from build123d import *

# Parameters (mm, degrees)
BOSS_EXTRUDE1_DEPTH = 17
M8_TAPPED_HOLE1_D   = 6.8


with BuildPart() as part:
    # Sketch1 → Boss-Extrude1 (new body)
    with BuildSketch(Plane(origin=(0, 0, 0), x_dir=(1, 0, 0), z_dir=(0, 1, 0))):
        with BuildLine():
            Line((10.214282758, -18.266545266), (13.128495977, -15.352332485))
            ThreePointArc((13.128495977, -15.352332485), (13.345268844, -15.027908548), (13.421388977, -14.645224485))
            Line((13.421388977, -14.645224485), (13.421388977, -5.451641485))
            ThreePointArc((13.421388977, -5.451641485), (13.345268461, -5.068958498), (13.128495977, -4.744535485))
            Line((13.128495977, -4.744535485), (10.214282758, -1.830320704))
            ThreePointArc((10.214282758, -1.830320704), (9.889859409, -1.613547953), (9.507175977, -1.537427485))
            Line((9.507175977, -1.537427485), (8.421388977, -1.537427485))
            ThreePointArc((8.421388977, -1.537427485), (7.714282177, -1.830320722), (7.421388977, -2.537427537))
            Line((7.421388977, -2.537427537), (7.421388977, -5.159438485))
            Line((7.421388977, -5.159438485), (4.421388977, -5.159438485))
            Line((4.421388977, -5.159438485), (4.421388977, -14.959438485))
            Line((4.421388977, -14.959438485), (7.421388977, -14.959438485))
            Line((7.421388977, -14.959438485), (7.421388977, -17.559438537))
            ThreePointArc((7.421388977, -17.559438537), (7.714282276, -18.266545347), (8.421389151, -18.559438485))
            Line((8.421389151, -18.559438485), (9.507176151, -18.559438485))
            ThreePointArc((9.507176151, -18.559438485), (9.88985949, -18.483317984), (10.214282758, -18.266545266))
        make_face()
    extrude(amount=BOSS_EXTRUDE1_DEPTH)

    # M8 Tapped Hole1 (through all)
    with Locations(Plane(origin=(4.421388977, 8.5, 10.059438485), x_dir=(0, 0, -1), z_dir=(-1, 0, 0))):
        with Locations((0, 0)):
            Hole(M8_TAPPED_HOLE1_D / 2)


solid = part.part
Design review of the part built by this model. Coordinates are the model's own, in mm. A direction names the side the tool comes from. Round coordinates to 2 decimals unless told otherwise and drop trailing zeros. Write each loop counter-clockwise with the first axis right and the second up, starting at its lowest first coordinate (ties: lowest second). Pieces come first, ordered by that corner, then holes. Notation, with made-up numbers: (10, -2.5) - (28, -2.5) arc R6 ccw to (28, 6.5) - close; hole circle Ø8 at (59.5, 31). An arc over 180 degrees is marked (long way). Use a Markdown table: item, result. Add a question column.
1. Clearance check with flat-ended pins moving along their axes: pin 1 (2 mm diameter, centred on y = 7, z = 4.5, fed in from -X); pin 2 (0.8 mm diameter, centred on y = 5, z = 16, fed in from -X); pin 3 (1.5 mm diameter, centred on x = 12.5, y = 8, fed in from -Z); pin 4 (1.5 mm diameter, centred on x = 6, y = 12, fed in from -Z). State where each tip first meets the part, or that it passes through.
2. We need section A-A (y = 8.5). State the section outline as (x, z) points, then the cut area to 3 significant figures.
3. We need section D-D (y = 12.75). State the section outline as (x, z) points.
4. For faces 1 (the face through (7.421, 8, 16)), 2 (the face through (7.421, 8, 4)), 3 (the face through (9, 8, 1.537)), list the 3-axis set-ups (+Z, -Z, +X, -X, +Y, -Y) from which the entire face can be reached by the end or side of a thin tool; tool diameter is ignored.
5. We need section B-B (x = 5.5). State the section outline as (y, z) points.
6. Wall thickness on probe 1 along Z at (x, y) = (6.75, 8.5); probe 2 along Z at (x, y) = (9.25, 8.5); probe 3 along Y at (x, z) = (11, 12.75): over which ranges is each line inside the solid? List them lowest first.
7. Mouldability with a two-part tool opening along Y and no side actions: class faces 4 (the face through (9, 9.8, 13.2)), 5 (the face through (9, 17, 10)), 6 (the face through (9, 0, 10)), 7 (the face through (11.65, 8.38, 16.83)) as +Y half, -Y half, draft (parallel to the pull), parting line (faces both ways), or undercut.
8. We need section C-C (z = 12.5). State the section outline as (x, y) points, then the cut area to 3 significant figures.
Output:
| question | item | result |
|---|---|---|
| 1 | pin 1 | stops at x = 4.42 |
| 1 | pin 2 | stops at x = 7.42 |
| 1 | pin 3 | stops at z = 3.37 |
| 1 | pin 4 | stops at z = 5.16 |
| 2 | outline | (4.42, 5.16) - (7.42, 5.16) - (7.42, 2.54) arc R1 ccw to (8.42, 1.54) - (9.51, 1.54) arc R1 ccw to (10.21, 1.83) - (13.13, 4.74) arc R1 ccw to (13.42, 5.45) - (13.42, 6.66) - (4.42, 6.66) - close; (4.42, 13.46) - (13.42, 13.46) - (13.42, 14.65) arc R1 ccw to (13.13, 15.35) - (10.21, 18.27) arc R1 ccw to (9.51, 18.56) - (8.42, 18.56) arc R1 ccw to (7.42, 17.56) - (7.42, 14.96) - (4.42, 14.96) - close |
| 2 | area | 57.6 mm2 |
| 3 | outline | (4.42, 5.16) - (7.42, 5.16) - (7.42, 2.54) arc R1 ccw to (8.42, 1.54) - (9.51, 1.54) arc R1 ccw to (10.21, 1.83) - (13.13, 4.74) arc R1 ccw to (13.42, 5.45) - (13.42, 14.65) arc R1 ccw to (13.13, 15.35) - (10.21, 18.27) arc R1 ccw to (9.51, 18.56) - (8.42, 18.56) arc R1 ccw to (7.42, 17.56) - (7.42, 14.96) - (4.42, 14.96) - close |
| 4 | face 1 | +Z, -X, +Y, -Y |
| 4 | face 2 | -Z, -X, +Y, -Y |
| 4 | face 3 | -Z, +X, -X, +Y, -Y |
| 5 | outline | (0, 5.16) - (17, 5.16) - (17, 14.96) - (0, 14.96) - close; hole circle Ø6.8 at (8.5, 10.06) |
| 6 | probe 1 | z = 5.16 to 6.66, 13.46 to 14.96 |
| 6 | probe 2 | z = 1.54 to 6.66, 13.46 to 18.56 |
| 6 | probe 3 | y = 0 to 6.42, 10.58 to 17 |
| 7 | face 4 | undercut |
| 7 | face 5 | +Y half |
| 7 | face 6 | -Y half |
| 7 | face 7 | draft |
| 8 | outline | (4.42, 0) - (13.42, 0) - (13.42, 6.13) - (4.42, 6.13) - close; (4.42, 10.87) - (13.42, 10.87) - (13.42, 17) - (4.42, 17) - close |
| 8 | area | 110 mm2 |
